from build123d import *

# Parameters (mm, degrees)
BOSS_EXTRUDE1_DEPTH  = 2
M3_CLEARANCE_HOLE1_D = 3.2
SKETCH4_W            = 35
SKETCH4_H            = 22
SKETCH4_W_2          = 22
SKETCH4_H_2          = 35
CUT_EXTRUDE1_DEPTH   = 96.480364474
FILLET1_R            = 3


with BuildPart() as part:
    # Sketch1 → Boss-Extrude1 (new body)
    with BuildSketch(Plane(origin=(0, 0, 0), x_dir=(1, 0, 0), z_dir=(0, 1, 0))):
        Polygon((-42.751262658, 67.5), (-67.5, 42.751262658), (-67.5, -42.751262658), (-42.751262658, -67.5), (42.751262658, -67.5), (67.5, -42.751262658), (67.5, 42.751262658), (42.751262658, 67.5), align=None)
    extrude(amount=BOSS_EXTRUDE1_DEPTH)

    # M3 Clearance Hole1 (through all)
    with Locations(Plane(origin=(0, 2, 0), x_dir=(1, 0, 0), z_dir=(0, 1, 0))):
        with Locations((-35, 60), (35, -60), (35, 60), (-35, -60)):
            Hole(M3_CLEARANCE_HOLE1_D / 2)

    # Sketch4 → Cut-Extrude1 (cut, through all)
    with BuildSketch(Plane(origin=(0, 2, 0), x_dir=(1, 0, 0), z_dir=(0, 1, 0))):
        with Locations((0, 45)):
            Rectangle(SKETCH4_W, SKETCH4_H)
        with Locations((-50, 0)):
            Rectangle(SKETCH4_W_2, SKETCH4_H_2)
        with Locations((50, 0)):
            Rectangle(SKETCH4_W_2, SKETCH4_H_2)
        with Locations((0, -45)):
            Rectangle(SKETCH4_W, SKETCH4_H)
    extrude(amount=-CUT_EXTRUDE1_DEPTH, mode=Mode.SUBTRACT)

    # Fillet1
    fillet1_edges = [part.edges().sort_by_distance(p)[0] for p in [
        (-17.5, 1, -34),
        (-17.5, 1, -56),
        (17.5, 1, -56),
        (17.5, 1, -34),
        (-39, 1, -17.5),
        (-39, 1, 17.5),
        (-61, 1, 17.5),
        (-61, 1, -17.5),
        (61, 1, -17.5),
        (61, 1, 17.5),
        (39, 1, 17.5),
        (39, 1, -17.5),
        (17.5, 1, 34),
        (17.5, 1, 56),
        (-17.5, 1, 56),
        (-17.5, 1, 34),
    ]]
    fillet(fillet1_edges, radius=FILLET1_R)


solid = part.part
Check sheet for the modelled part. Datum: model origin and axes. Units: mm. A direction names the side the tool comes from. Round coordinates to 2 decimals unless told otherwise and drop trailing zeros. Order: outer loops, then holes, each group sorted by start corner. A loop starts at its lowest first (then second) coordinate and runs counter-clockwise, first axis right, second up.
(1) Draft check along X on faces 1 (the cylindrical face through (-39.9, 0.99, 16.64)), 2 (the flat face through (-54.95, 0.99, -55.3)), 3 (the flat face through (-1, 2, -1)). Enter one of: pulls with the +X half, pulls with the -X half, needs draft (parallel to the pull), parting line crosses it, or undercut.
(2) Go/stop test with flat-tipped pins: P1, Ø2.5, axis at x = 35, z = -60, coming from the -Y side; P2, Ø0.6, axis at y = 0.5, z = 45.5, coming from the +X side; P3, Ø0.6, axis at x = -52, y = 1, coming from the +Z side; P4, Ø1, axis at x = -48.5, y = 1, coming from the -Z side. Record where each tip stops, or that it passes through.
(3) Cross-section at A-A, the plane z = -10.5. Enter the section's corners in (x, y), and give its area (3 significant figures).
(4) Scan lines: probe 1 along Z at (x, y) = (-2, 1.8); probe 2 along Z at (x, y) = (35, 0.65); probe 3 along X at (y, z) = (0.3, -2.5). Record each from-to range of solid material in increasing order.
(5) Access from +Z, -Z, +X, -X, +Y, -Y to the whole of each face (thin tool, end or side, straight path). Record for faces 4 (the cylindrical face through (-60.1, 0.99, -16.64)), 5 (the flat face through (-1, 0, -1)).
(6) Cross-section at B-B, the plane x = -54.5. Enter the section's corners in (y, z), and give its area (3 significant figures).
(7) Cross-section at C-C, the plane x = -35. Enter the section's corners in (y, z), and give its area (3 significant figures).
(8) Cross-section at D-D, the plane y = 0.95. State how many separate pieces and enclosed holes the cut face has, and give its area (3 significant figures).
Check sheet entries:
1. face 1: undercut
1. face 2: pulls with the -X half
1. face 3: needs draft
2. P1: passes through
2. P2: stops at x = 65.05
2. P3: stops at z = 58.55
2. P4: stops at z = -62.25
3. outline: (-67.5, 0) - (-61, 0) - (-61, 2) - (-67.5, 2) - close; (-39, 0) - (39, 0) - (39, 2) - (-39, 2) - close; (61, 0) - (67.5, 0) - (67.5, 2) - (61, 2) - close
3. area: 182 mm2
4. probe 1: z = -67.5 to -56, -34 to 34, 56 to 67.5
4. probe 2: z = -67.5 to -61.6, -58.4 to 58.4, 61.6 to 67.5
4. probe 3: x = -67.5 to -61, -39 to 39, 61 to 67.5
5. face 4: +Y, -Y
5. face 5: +Z, -Z, +X, -X, -Y
6. outline: (0, -55.75) - (2, -55.75) - (2, -17.5) - (0, -17.5) - close; (0, 17.5) - (2, 17.5) - (2, 55.75) - (0, 55.75) - close
6. area: 153 mm2
7. outline: (0, -67.5) - (2, -67.5) - (2, -61.6) - (0, -61.6) - close; (0, -58.4) - (2, -58.4) - (2, 58.4) - (0, 58.4) - close; (0, 61.6) - (2, 61.6) - (2, 67.5) - (0, 67.5) - close
7. area: 257 mm2
8. separate pieces: 1
8. enclosed holes: 8
8. area: 13,900 mm2
